Autodesk Inventor part; units mm, degrees
ref_plane "YZ Plane" through (0, 0, 0) normal (1, 0, 0) x (0, 1, 0)
ref_plane "XZ Plane" through (0, 0, 0) normal (0, 1, 0) x (-1, 0, 0)
ref_plane "XY Plane" through (0, 0, 0) normal (0, 0, 1) x (1, 0, 0)
sketch "Sketch1" plane through (0, 0, 0) normal (0, 0, 1) x (1, 0, 0)
  arc A0 (-15, -160) -> (0, -175) centre (0, -160) ccw
  line L0 (0, 15) -> (160, 15)
  line L1 (175, 0) -> (175, -160)
  line L2 (160, -175) -> (0, -175)
  line L3 (-15, -160) -> (-15, 0)
  arc A1 (0, 15) -> (-15, 0) centre (0, 0) ccw
  arc A2 (160, -175) -> (175, -160) centre (160, -160) ccw
  arc A3 (175, 0) -> (160, 15) centre (160, 0) ccw
  point P0 (-15, 15)
  dimension "d0" = 190
  dimension "d1" = 190
  dimension "d2" = 15
extrude "Extrusion1" add sketch "Sketch1" along normal blind 12.7
sketch "Sketch2" plane through (0, 0, 12.7) normal (0, 0, 1) x (1, 0, 0)
  line L0 (-15, 0) -> (-15, -160)
  arc A0 (-15, -160) -> (0, -175) centre (0, -160) ccw
  line L1 (0, -175) -> (160, -175)
  arc A1 (160, -175) -> (175, -160) centre (160, -160) ccw
  line L2 (175, -160) -> (175, 0)
  arc A2 (175, 0) -> (160, 15) centre (160, 0) ccw
  line L3 (160, 15) -> (0, 15)
  arc A3 (0, 15) -> (-15, 0) centre (0, 0) ccw
  line L4 (0, 0) -> (160, -160) construction
  line L5 (147.3, -152.3) -> (12.7, -152.3)
  line L6 (7.7, -147.3) -> (7.7, -12.7)
  line L7 (12.7, -7.7) -> (147.3, -7.7)
  line L8 (152.3, -12.7) -> (152.3, -147.3)
  line L9 (152.3, -152.3) -> (7.7, -7.7) construction
  line L10 (7.7, -152.3) -> (152.3, -7.7) construction
  arc A4 (12.7, -7.7) -> (7.7, -12.7) centre (12.7, -12.7) ccw
  arc A5 (152.3, -12.7) -> (147.3, -7.7) centre (147.3, -12.7) ccw
  arc A6 (147.3, -152.3) -> (152.3, -147.3) centre (147.3, -147.3) ccw
  arc A7 (7.7, -147.3) -> (12.7, -152.3) centre (12.7, -147.3) ccw
  line L11 (147.3, 5) -> (12.7, 5)
  arc A8 (12.7, 5) -> (-5, -12.7) centre (12.7, -12.7) ccw
  line L12 (-5, -12.7) -> (-5, -147.3)
  arc A9 (-5, -147.3) -> (12.7, -165) centre (12.7, -147.3) ccw
  line L13 (12.7, -165) -> (147.3, -165)
  arc A10 (147.3, -165) -> (165, -147.3) centre (147.3, -147.3) ccw
  line L14 (165, -147.3) -> (165, -12.7)
  arc A11 (165, -12.7) -> (147.3, 5) centre (147.3, -12.7) ccw
  point P0 (80, -80)
  dimension "d7" = 5
  dimension "d8" = 12.7
  dimension "d9" = 10
extrude "Extrusion2" cut sketch "Sketch2" against normal blind 7 contours A11 L14 A10 L13 A9 L12 A8 L11
sketch "Sketch3" plane through (0, 0, 0) normal (0, 0, -1) x (-1, 0, 0)
  line L0 (-140, -10.675) -> (-20, -10.675) construction
  line L1 (-147.3, -7.7) -> (-12.7, -7.7)
  line L2 (-140, -13.85) -> (-20, -13.85)
  line L3 (-20, -7.5) -> (-140, -7.5)
  arc A0 (-140, -7.5) -> (-140, -13.85) centre (-140, -10.675) ccw
  arc A1 (-20, -13.85) -> (-20, -7.5) centre (-20, -10.675) ccw
  line L4 (15, -160) -> (15, 0)
  line L5 (-175, 0) -> (-175, -160)
  arc A2 (-160, 15) -> (-175, 0) centre (-160, 0) ccw
  arc A3 (0, -175) -> (15, -160) centre (0, -160) ccw
  line L6 (-160, 0) -> (0, -160) construction
  circle A4 centre (-80, -80) radius 16.0572 construction
  arc A5 (-152.5, -140) -> (-146.15, -140) centre (-149.325, -140) ccw
  line L7 (-152.5, -20) -> (-152.5, -140)
  line L8 (-146.15, -140) -> (-146.15, -20)
  arc A6 (-146.15, -20) -> (-152.5, -20) centre (-149.325, -20) ccw
  line L9 (-149.325, -140) -> (-149.325, -20) construction
  arc A7 (-20, -152.5) -> (-20, -146.15) centre (-20, -149.325) ccw
  line L10 (-140, -152.5) -> (-20, -152.5)
  line L11 (-20, -146.15) -> (-140, -146.15)
  arc A8 (-140, -146.15) -> (-140, -152.5) centre (-140, -149.325) ccw
  line L12 (-20, -149.325) -> (-140, -149.325) construction
  arc A9 (-7.5, -20) -> (-13.85, -20) centre (-10.675, -20) ccw
  line L13 (-7.5, -140) -> (-7.5, -20)
  line L14 (-13.85, -20) -> (-13.85, -140)
  arc A10 (-13.85, -140) -> (-7.5, -140) centre (-10.675, -140) ccw
  line L15 (-10.675, -20) -> (-10.675, -140) construction
  point P0 (0, 0)
  point P1 (-80, -10.675)
  point P2 (-149.325, -80)
  point P3 (-80, -149.325)
  point P4 (-10.675, -80)
  dimension "d12" = 6.35
  dimension "d13" = 0.2
  dimension "d14" = 35
  dimension "d15" = 35
  dimension "d18" = 360
extrude "Extrusion3" cut sketch "Sketch3" against normal blind 8
sketch "Sketch4" plane through (0, 0, 0) normal (0, 0, -1) x (-1, 0, 0)
  arc A0 (0, -175) -> (15, -160) centre (0, -160) ccw
  arc A1 (-160, 15) -> (-175, 0) centre (-160, 0) ccw
  line L0 (0, -160) -> (-160, 0) construction
  line L1 (-2, 11.5) -> (-158, 11.5)
  line L2 (-171.5, -2) -> (-171.5, -158)
  line L3 (-158, -171.5) -> (-2, -171.5)
  line L4 (11.5, -158) -> (11.5, -2)
  line L5 (11.5, 11.5) -> (-171.5, -171.5) construction
  line L6 (-171.5, 11.5) -> (11.5, -171.5) construction
  arc A2 (-2, -171.5) -> (11.5, -158) centre (-2, -158) ccw
  arc A3 (-171.5, -158) -> (-158, -171.5) centre (-158, -158) ccw
  arc A4 (-158, 11.5) -> (-171.5, -2) centre (-158, -2) ccw
  arc A5 (11.5, -2) -> (-2, 11.5) centre (-2, -2) ccw
  arc A6 (-20, -152.5) -> (-20, -146.15) centre (-20, -149.325) ccw
  line L7 (-20, -152.5) -> (-140, -152.5)
  arc A7 (-140, -146.15) -> (-140, -152.5) centre (-140, -149.325) ccw
  line L8 (-140, -146.15) -> (-20, -146.15)
  arc A8 (-20, -13.85) -> (-20, -7.5) centre (-20, -10.675) ccw
  line L9 (-20, -13.85) -> (-140, -13.85)
  arc A9 (-140, -7.5) -> (-140, -13.85) centre (-140, -10.675) ccw
  line L10 (-140, -7.5) -> (-20, -7.5)
  arc A10 (-152.5, -140) -> (-146.15, -140) centre (-149.325, -140) ccw
  line L11 (-152.5, -140) -> (-152.5, -20)
  arc A11 (-146.15, -20) -> (-152.5, -20) centre (-149.325, -20) ccw
  line L12 (-146.15, -20) -> (-146.15, -140)
  arc A12 (-7.5, -20) -> (-13.85, -20) centre (-10.675, -20) ccw
  line L13 (-7.5, -20) -> (-7.5, -140)
  arc A13 (-13.85, -140) -> (-7.5, -140) centre (-10.675, -140) ccw
  line L14 (-13.85, -140) -> (-13.85, -20)
  line L15 (15, -160) -> (15, 0)
  arc A14 (15, 0) -> (0, 15) centre (0, 0) ccw
  line L16 (0, 15) -> (-160, 15)
  arc A15 (-160, 15) -> (-175, 0) centre (-160, 0) ccw
  line L17 (-175, 0) -> (-175, -160)
  arc A16 (-175, -160) -> (-160, -175) centre (-160, -160) ccw
  line L18 (-160, -175) -> (0, -175)
  arc A17 (0, -175) -> (15, -160) centre (0, -160) ccw
  point P0 (-80, -80)
  dimension "d22" = 183
  dimension "d23" = 183
  dimension "d24" = 13.5
extrude "Extrusion4" cut sketch "Sketch4" against normal blind 9 contours L18 A16 L17 A1 L16 A14 L15 A0
equation "\"d14\" = d15"
properties part number "NewLid"
Here's how the part is built. I have some questions about the finished solid (model axes, mm). A direction names the side the tool comes from. Give positions to 0.01 mm unless a question says otherwise; leave off trailing zeros. Loops run counter-clockwise (first coordinate to the right, second up) from the corner with the lowest first, then second, coordinate; pieces in that order, holes last. Notation, with made-up numbers: M -38,12 L -7,12 A19 ccw -7,45 Z; hole C -24.75,47.5 d7. An arc over 180 degrees is marked long. Return JSON: item names as keys, results as strings.
Item 1: Please list where these lines run through material, in increasing order: line 1 (Y direction, x = 48.5, z = 3.5); line 2 (X direction, y = -98.5, z = 3); line 3 (X direction, y = -146, z = 11.5).
A:
{"line 1": "y = -171.5 to -152.5, -146.15 to -13.85, -7.5 to 11.5", "line 2": "x = -11.5 to 7.5, 13.85 to 146.15, 152.5 to 171.5", "line 3": "x = -15 to -5, 7.7 to 152.3, 165 to 175"}
Item 2: On a 3-axis mill with a long thin cutter (end or side, diameter ignored), from which of +Z, -Z, +X, -X, +Y, -Y can I reach the whole of each face in a straight line? I mean faces 5 (the flat face through (79, -146.15, 4)), 6 (the cylindrical face through (159.95, -0.32, 9.25)), 7 (the flat face through (81, -171.5, 4)). Say none if no direction works.
A:
{"face 5": "-Z", "face 6": "+Z", "face 7": "-Z, +X, -X, -Y"}
Item 3: I'm going to push flat-ended pins straight in: pin 1 Ø4.5 at (y, z) = (-69.5, 3) entering from +X; pin 2 Ø1.8 at (x, y) = (12, -99.5) entering from -Z; pin 3 Ø6.5 at (y, z) = (-63, 2) entering from -X. Where does each tip first touch, or does it pass through?
A:
{"pin 1": "stops at x = 171.5", "pin 2": "stops at z = 8", "pin 3": "stops at x = -11.5"}
Item 4: Imagine slicing it at C-C on z = 2. List the corners of the cut face in (x, y) for me (3 decimals).
A:
{"outline": "M -11.5,-158 A13.5 ccw 2,-171.5 L 158,-171.5 A13.5 ccw 171.5,-158 L 171.5,-2 A13.5 ccw 158,11.5 L 2,11.5 A13.5 ccw -11.5,-2 Z; hole M 7.5,-140 A3.175 ccw 13.85,-140 L 13.85,-20 A3.175 ccw 7.5,-20 Z; hole M 20,-152.5 L 140,-152.5 A3.175 ccw 140,-146.15 L 20,-146.15 A3.175 ccw Z; hole M 20,-13.85 L 140,-13.85 A3.175 ccw 140,-7.5 L 20,-7.5 A3.175 ccw Z; hole M 146.15,-140 A3.175 ccw 152.5,-140 L 152.5,-20 A3.175 ccw 146.15,-20 Z"}
Item 5: Imagine slicing it at B-B on y = -112. List the corners of the cut face in (x, z) for me, then the cut area to 3 significant figures.
A:
{"outline": "M -15,9 L -11.5,9 L -11.5,0 L 7.5,0 L 7.5,5.7 L -5,5.7 L -5,12.7 L -15,12.7 Z; M 7.7,8 L 13.85,8 L 13.85,0 L 146.15,0 L 146.15,8 L 152.3,8 L 152.3,12.7 L 7.7,12.7 Z; M 152.5,0 L 171.5,0 L 171.5,9 L 175,9 L 175,12.7 L 165,12.7 L 165,5.7 L 152.5,5.7 Z", "area": "2,070 mm^2"}
Item 6: Thinking about a two-plate mould opening in Y: for faces 1 (the flat face through (152.5, -79, 3)), 2 (the cylindrical face through (-7.65, 7.44, 4.44)), 3 (the cylindrical face through (0.32, -0.05, 9.25)), 4 (the flat face through (123, 12, 9)), which applies, released by +Y, released by -Y, zero draft, split by the parting line, or undercut?
A:
{"face 1": "undercut", "face 2": "released by +Y", "face 3": "undercut", "face 4": "zero draft"}
Item 7: Imagine slicing it at A-A on x = 92.5. List the corners of the cut face in (y, z) for me, then the cut area to 3 significant figures.
A:
{"outline": "M -175,9 L -171.5,9 L -171.5,0 L -152.5,0 L -152.5,5.7 L -165,5.7 L -165,12.7 L -175,12.7 Z; M -152.3,8 L -146.15,8 L -146.15,0 L -13.85,0 L -13.85,8 L -7.7,8 L -7.7,12.7 L -152.3,12.7 Z; M -7.5,0 L 11.5,0 L 11.5,9 L 15,9 L 15,12.7 L 5,12.7 L 5,5.7 L -7.5,5.7 Z", "area": "2,070 mm^2"}
Item 8: Imagine slicing it at D-D on x = 5. List the corners of the cut face in (y, z) for me, then the cut area to 3 significant figures.
A:
{"outline": "M -175,9 L -171.5,9 L -171.5,0 L 11.5,0 L 11.5,9 L 15,9 L 15,12.7 L 3.24,12.7 L 3.24,5.7 L -163.24,5.7 L -163.24,12.7 L -175,12.7 Z", "area": "1,180 mm^2"}
